```python
from build123d import *

# Parameters (mm, degrees)
SKETCH_1_W      = 119.4
SKETCH_1_H      = 59.4
SKETCH_1_R      = 3
EXTRUDE_1_DEPTH = 4
FILLET_1_R      = 7


with BuildPart() as part:
    # Эскиз1 → Бобышка-Вытянуть1 (new body)
    with BuildSketch(Plane.XY):
        Rectangle(SKETCH_1_W, SKETCH_1_H)
        with Locations((0, -13.97221548)):
            Circle(SKETCH_1_R, mode=Mode.SUBTRACT)
        with BuildLine():
            Line((3.25, 10.5), (3.25, -10.5))
            ThreePointArc((3.25, -10.5), (14, -16), (24.75, -10.5))
            Line((24.75, -10.5), (24.75, 10.5))
            ThreePointArc((24.75, 10.5), (14, 16), (3.25, 10.5))
        make_face(mode=Mode.SUBTRACT)
        with BuildLine():
            Line((48.25, 10.5), (48.25, -10.5))
            ThreePointArc((48.25, -10.5), (37.5, -16), (26.75, -10.5))
            Line((26.75, -10.5), (26.75, 10.5))
            ThreePointArc((26.75, 10.5), (37.5, 16), (48.25, 10.5))
        make_face(mode=Mode.SUBTRACT)
        with BuildLine():
            Line((-26.75, 10.5), (-26.75, -10.5))
            ThreePointArc((-26.75, -10.5), (-37.5, -16), (-48.25, -10.5))
            Line((-48.25, -10.5), (-48.25, 10.5))
            ThreePointArc((-48.25, 10.5), (-37.5, 16), (-26.75, 10.5))
        make_face(mode=Mode.SUBTRACT)
        with BuildLine():
            Line((-3.25, 10.5), (-3.25, -10.5))
            ThreePointArc((-3.25, -10.5), (-14, -16), (-24.75, -10.5))
            Line((-24.75, -10.5), (-24.75, 10.5))
            ThreePointArc((-24.75, 10.5), (-14, 16), (-3.25, 10.5))
        make_face(mode=Mode.SUBTRACT)
    extrude(amount=EXTRUDE_1_DEPTH)

    # Скругление1
    fillet_1_edges = [part.edges().sort_by_distance(p)[0] for p in [
        (59.7, -29.7, 2),
        (-59.7, -29.7, 2),
        (-59.7, 29.7, 2),
        (59.7, 29.7, 2),
    ]]
    fillet(fillet_1_edges, radius=FILLET_1_R)


solid = part.part
```
For this review, take the finished solid that the model builds, in its own axes (mm). A direction names the side the tool comes from. Give positions to 0.01 mm unless a question says otherwise; leave off trailing zeros. Order: outer loops, then holes, each group sorted by start corner. A loop starts at its lowest first (then second) coordinate and runs counter-clockwise, first axis right, second up.
1) For faces 1 (the face through (-26.75, 0, 2)), 2 (the face through (-59.7, 0, 2)), list the 3-axis set-ups (+Z, -Z, +X, -X, +Y, -Y) from which the entire face can be reached by the end or side of a thin tool; tool diameter is ignored.
2) The part is to be moulded in two halves that separate along Y. For faces 3 (the face through (-1, 29.7, 2)), 4 (the face through (-3.25, 0, 2)), 5 (the face through (-1, 0, 0)), say which applies: released by +Y, released by -Y, zero draft, split by the parting line, or undercut.
3) Take a section at C-C (z = 1.85). Give the boundary of the cut face in (x, y), then the cut area to 3 significant figures.
4) Insertion check: pin 1 (8 mm diameter, centred on x = 1.5, y = 17, fed in from -Z). The pin has a flat end and moves straight along its axis. Give the tip position at first contact, or say it passes through.
5) Take a section at A-A (x = 0). Give the boundary of the cut face in (y, z).
6) Wall thickness on line 1 (X direction, y = 6.5, z = 1.5); line 2 (Y direction, x = 0, z = 1.55): over which ranges is each line inside the solid? List them lowest first.
7) Take a section at B-B (y = -8). Give the boundary of the cut face in (x, z), then the cut area to 3 significant figures.
8) Take a section at D-D (x = 21). Give the boundary of the cut face in (y, z), then the cut area to 3 significant figures.
Derived:
1. face 1: +Z, -Z
1. face 2: +Z, -Z, -X, +Y, -Y
2. face 3: released by +Y
2. face 4: undercut
2. face 5: zero draft
3. outline: (-59.7, -22.7) arc R7 ccw to (-52.7, -29.7) - (52.7, -29.7) arc R7 ccw to (59.7, -22.7) - (59.7, 22.7) arc R7 ccw to (52.7, 29.7) - (-52.7, 29.7) arc R7 ccw to (-59.7, 22.7) - close; hole (-48.25, -10.5) arc R13.26 ccw to (-26.75, -10.5) - (-26.75, 10.5) arc R13.26 ccw to (-48.25, 10.5) - close; hole (-24.75, -10.5) arc R13.26 ccw to (-3.25, -10.5) - (-3.25, 10.5) arc R13.26 ccw to (-24.75, 10.5) - close; hole circle Ø6 at (0, -13.97); hole (3.25, -10.5) arc R13.26 ccw to (24.75, -10.5) - (24.75, 10.5) arc R13.26 ccw to (3.25, 10.5) - close; hole (26.75, -10.5) arc R13.26 ccw to (48.25, -10.5) - (48.25, 10.5) arc R13.26 ccw to (26.75, 10.5) - close
3. area: 4,550 mm2
4. pin 1: stops at z = 0
5. outline: (-29.7, 0) - (-16.97, 0) - (-16.97, 4) - (-29.7, 4) - close; (-10.97, 0) - (29.7, 0) - (29.7, 4) - (-10.97, 4) - close
6. line 1: x = -59.7 to -48.25, -26.75 to -24.75, -3.25 to 3.25, 24.75 to 26.75, 48.25 to 59.7
6. line 2: y = -29.7 to -16.97, -10.97 to 29.7
7. outline: (-59.7, 0) - (-48.25, 0) - (-48.25, 4) - (-59.7, 4) - close; (-26.75, 0) - (-24.75, 0) - (-24.75, 4) - (-26.75, 4) - close; (-3.25, 0) - (3.25, 0) - (3.25, 4) - (-3.25, 4) - close; (24.75, 0) - (26.75, 0) - (26.75, 4) - (24.75, 4) - close; (48.25, 0) - (59.7, 0) - (59.7, 4) - (48.25, 4) - close
7. area: 134 mm2
8. outline: (-29.7, 0) - (-14, 0) - (-14, 4) - (-29.7, 4) - close; (14, 0) - (29.7, 0) - (29.7, 4) - (14, 4) - close
8. area: 126 mm2
